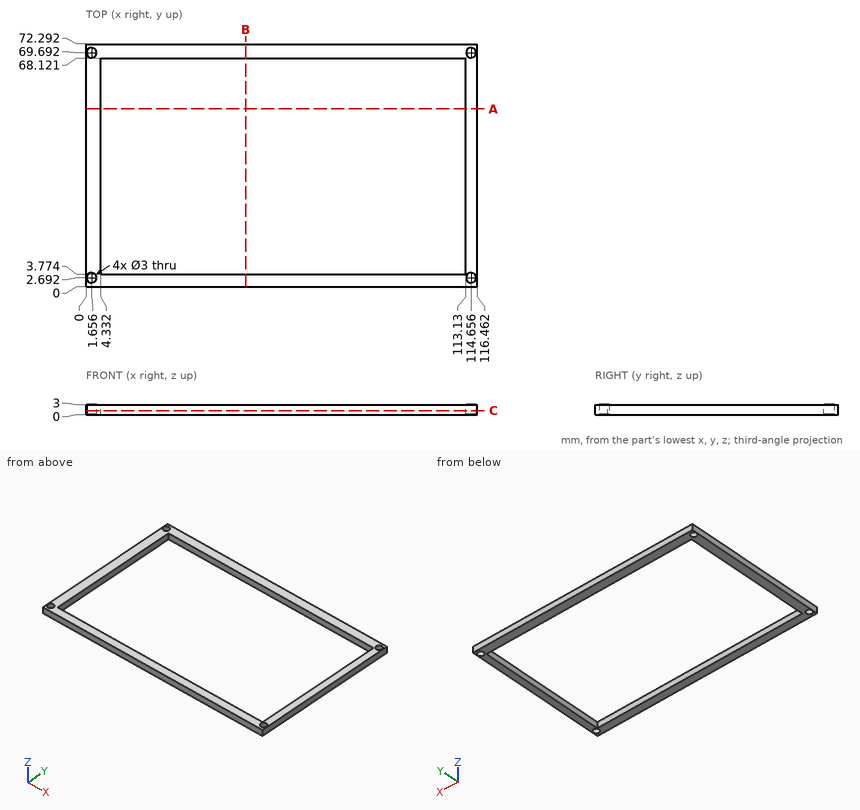
Geometry: see drawing. Coordinates: mm, zero at the bounding-box minimum. Round coordinates to 2 decimals unless told otherwise and drop trailing zeros. Write each loop counter-clockwise with the first axis right and the second up, starting at its lowest first coordinate (ties: lowest second). Pieces come first, ordered by that corner, then holes.
Item 1: Material intervals for L1, parallel to X at y = 14, z = 1.95; L2, parallel to Y at x = 66, z = 1.4; L3, parallel to X at y = 68.5, z = 1.2 (1 decimal), sorted ascending.
Item 2: Section query C-C (z = 1.3). Return loops of the section in (x, y).
Item 3: Section query A-A (y = 53). Return loops of the section in (x, z).
Item 4: Section query B-B (x = 47.5). Return loops of the section in (y, z).
Completed:
1. L1: x = 0 to 4.33, 113.13 to 116.46
1. L2: y = 0 to 3.77, 68.12 to 72.29
1. L3: x = 0 to 0.7, 2.6 to 113.7, 115.6 to 116.5
2. outline: (0, 0) - (116.46, 0) - (116.46, 72.29) - (0, 72.29) - close; hole circle Ø3 at (1.66, 2.69); hole circle Ø3 at (1.66, 69.69); hole (4.33, 3.77) - (113.13, 3.77) - (113.13, 68.12) - (4.33, 68.12) - close; hole circle Ø3 at (114.66, 2.69); hole circle Ø3 at (114.66, 69.69)
3. outline: (0, 0) - (4.33, 0) - (4.33, 3) - (0, 3) - close; (113.13, 0) - (116.46, 0) - (116.46, 3) - (113.13, 3) - close
4. outline: (0, 0) - (3.77, 0) - (3.77, 3) - (0, 3) - close; (68.12, 0) - (72.29, 0) - (72.29, 3) - (68.12, 3) - close
